Part model, mm, in its own coordinate system. Coordinates: 2 decimals unless noted, no trailing zeros. Write each loop counter-clockwise with the first axis right and the second up, starting at its lowest first coordinate (ties: lowest second). Pieces come first, ordered by that corner, then holes. Notation, with made-up numbers: M 64,-17.5 L 120,-17.5 A21 ccw 120,19.5 Z; hole C 64.5,-2.75 d11. An arc over 180 degrees is marked long. Use a Markdown table: item, result. Add a question column.
Q1. Wall check: L1, parallel to Z at x = -1, y = -0.5; L2, parallel to Y at x = 0, z = -14; L3, parallel to X at y = -1.75, z = -27. Give the ranges that are in metal, low to high. Write a range as from..to.
Q2. Pin check, flat tips, straight feed: pin 1 Ø4 at (x, y) = (1.5, -4) entering from -Z; pin 2 Ø1.5 at (x, z) = (-2.5, 27) entering from -Y; pin 3 Ø2 at (y, z) = (1.5, 2.5) entering from +X. Stop position of each tip, or through.
Q3. Slice it at B-B on z = -23.5. Write the cut outline in (x, y).
Q4. Slice it at A-A on y = 0. Write the cut outline in (x, z), then the cut area to 3 significant figures.
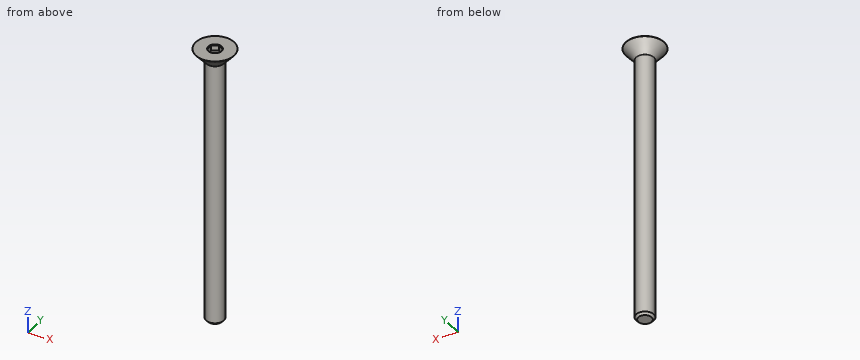
from build123d import *

# Parameters (mm, degrees)
SKETCH10_R         = 1.833087105
CUT_EXTRUDE2_DEPTH = 1.6129
CUT_EXTRUDE2_DRAFT = -45
CUT_EXTRUDE1_DEPTH = 1.6129


with BuildPart() as part:
    # Sketch2 → Revolve1 (revolve)
    with BuildSketch(Plane(origin=(0, 0, 0), x_dir=(0, 0, -1), z_dir=(1, 0, 0)), mode=Mode.PRIVATE) as revolve1_sk:
        with BuildLine():
            Line((-38.035484, 5.2197), (-34.8742, 2.471637744))
            ThreePointArc((-34.8742, 2.471637744), (-34.80108483, 2.428138789), (-34.717366229, 2.413))
            Line((-34.717366229, 2.413), (37.5046875, 2.413))
            Line((37.5046875, 2.413), (38.1, 1.8176875))
            Line((38.1, 1.8176875), (38.1, 0))
            Line((38.1, 0), (-38.1, 0))
            Line((-38.1, 0), (-38.1, 5.2197))
            Line((-38.1, 5.2197), (-38.035484, 5.2197))
        make_face()
    revolve(revolve1_sk.sketch.rotate(Axis((0, 0, -38.1), (0, 0, 1)), 90), axis=Axis((0, 0, -38.1), (0, 0, 1)))


with BuildPart() as cut_extrude2_tool:
    # Sketch10 → Cut-Extrude2 (with draft: the straight prism first)
    with BuildSketch(Plane.XY.offset(38.1)):
        Circle(SKETCH10_R)
    extrude(amount=-CUT_EXTRUDE2_DEPTH)
    # Cut-Extrude2: the draft: its side faces are tilted about the plane it starts from
    cut_extrude2_sides = [cut_extrude2_tool.faces().sort_by_distance(p)[0] for p in [
        (-1.833087105, 0, 37.29355),
    ]]
    draft(cut_extrude2_sides, Plane.XY.offset(38.1), CUT_EXTRUDE2_DRAFT)


with BuildPart() as part_1:
    add(part.part)

    # Cut-Extrude2: cut by cut_extrude2_tool
    add(cut_extrude2_tool.part, mode=Mode.SUBTRACT)

    # Sketch9 → Cut-Extrude1 (cut)
    with BuildSketch(Plane.XY.offset(38.1)):
        Polygon((1.5875, -0.916543552), (1.5875, 0.916543552), (0, 1.833087105), (-1.5875, 0.916543552), (-1.5875, -0.916543552), (0, -1.833087105), align=None)
    extrude(amount=-CUT_EXTRUDE1_DEPTH, mode=Mode.SUBTRACT)


solid = part_1.part
Recorded:
| question | item | result |
|---|---|---|
| 1 | L1 | -38.1..36.49 |
| 1 | L2 | -2.41..2.41 |
| 1 | L3 | -1.66..1.66 |
| 2 | pin 1 | z = -37.65 |
| 2 | pin 2 | y = -1.66 |
| 2 | pin 3 | x = 2.36 |
| 3 | outline | C 0,0 d4.83 |
| 4 | outline | M -5.22,38.04 L -2.47,34.87 A0.24 cw -2.41,34.72 L -2.41,-37.5 L -1.82,-38.1 L 1.82,-38.1 L 2.41,-37.5 L 2.41,34.72 A0.24 cw 2.47,34.87 L 5.22,38.04 L 5.22,38.1 L 1.83,38.1 L 1.59,37.85 L 1.59,36.49 L -1.59,36.49 L -1.59,37.85 L -1.83,38.1 L -5.22,38.1 Z |
| 4 | area | 372 mm² |
